Answer from the drawing. Dimensions are ordinates in mm from the lowest x, y and z of the part. A direction names the side the tool comes from. Give positions to 0.01 mm unless a question says otherwise; leave off trailing zeros. Order: outer loops, then holes, each group sorted by start corner. A loop starts at its lowest first (then second) coordinate and runs counter-clockwise, first axis right, second up. Notation, with made-up numbers: (72, 16.5) -> (119, 16.5) arc R16 cw to (119, 41.5) -> close; hole circle Ø4 at (59, 42.5). An arc over 180 degrees is marked (long way). Answer as a JSON object with one key per item and string values. Group by question number.
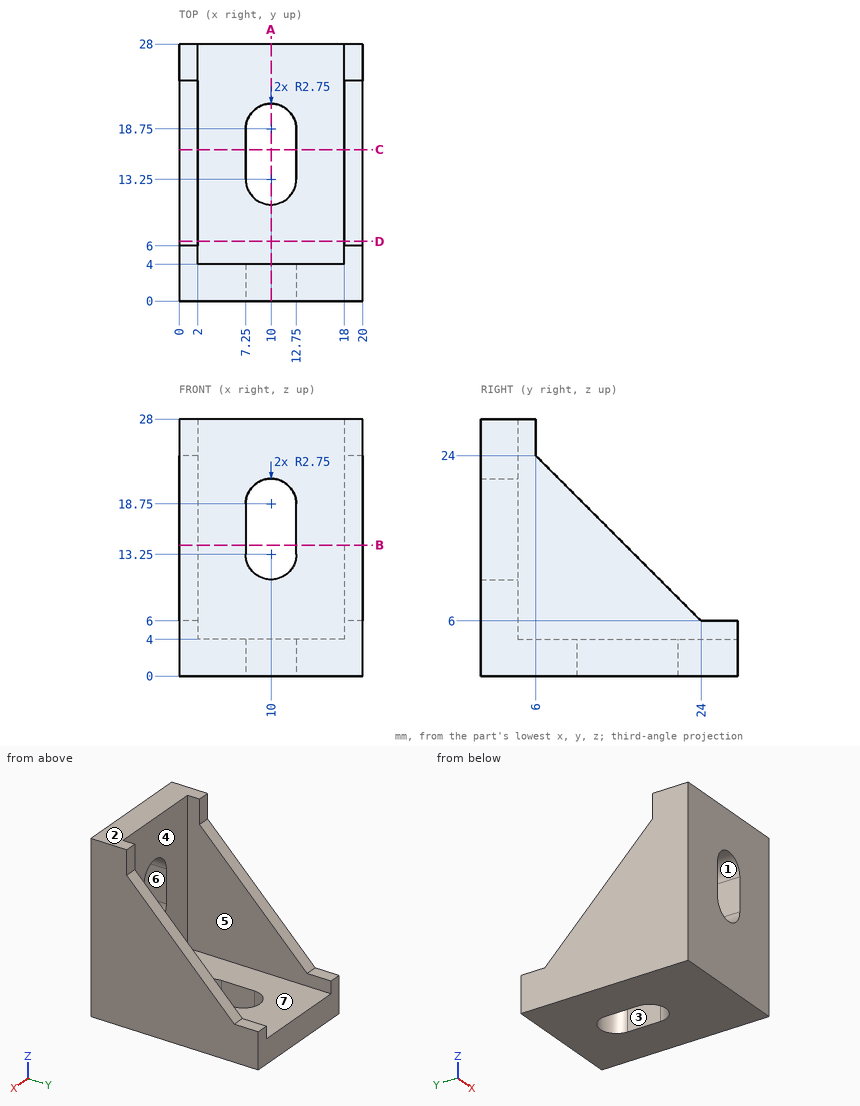
(1) A cutting plane is placed at B-B (z = 14.25). Determine the outline of the cut face in (x, y).
(2) Which of the six approach directions +Z, -Z, +X, -X, +Y, -Y give full straight-line access (tool end or side, diameter ignored) to the marked faces 1, 2, 3 and 4?
(3) Find the intervals of material crossed by line 1 along X through (y, z) = (6.5, 14); line 2 along Y through (x, z) = (5.25, 25.75), in increasing order. Write a range as [from, to].
(4) For a pull along Z with two mould halves and no side action, classify the marked faces 5, 6 and 7 as +Z half, -Z half, draft (parallel to the pull), parting line (faces both ways), or undercut.
(5) Flat-ended cylindrical pins translate along their axes: pin 1 Ø10 at (x, z) = (8, 22.5) entering from +Y; pin 2 Ø2 at (x, y) = (18.5, 25.5) entering from +Z; pin 3 Ø1 at (x, z) = (19, 27) entering from +Y. Find the tip coordinate at first contact, or state that the pin passes through.
(6) A cutting plane is placed at A-A (x = 10). Determine the outline of the cut face in (y, z).
(7) A cutting plane is placed at C-C (y = 16.5). Determine the outline of the cut face in (x, z), and give its area (3 significant figures).
(8) A cutting plane is placed at D-D (y = 6.5). Determine the outline of the cut face in (x, z), and give its area (3 significant figures).
Check sheet entries:
{
 "1": {"outline": "(0, 0) -> (7.25, 0) -> (7.25, 4) -> (2, 4) -> (2, 15.75) -> (0, 15.75) -> close; (12.75, 0) -> (20, 0) -> (20, 15.75) -> (18, 15.75) -> (18, 4) -> (12.75, 4) -> close"},
 "2": {"face 1": "+Y, -Y", "face 2": "+Z, +X, -X, +Y, -Y", "face 3": "+Z, -Z", "face 4": "+Z, +Y"},
 "3": {"line 1": "x = [0, 2], [18, 20]", "line 2": "y = [0, 4]"},
 "4": {"face 5": "draft", "face 6": "undercut", "face 7": "+Z half"},
 "5": {"pin 1": "stops at y = 4", "pin 2": "stops at z = 6", "pin 3": "stops at y = 6"},
 "6": {"outline": "(0, 0) -> (10.5, 0) -> (10.5, 4) -> (4, 4) -> (4, 10.5) -> (0, 10.5) -> close; (0, 21.5) -> (4, 21.5) -> (4, 28) -> (0, 28) -> close; (21.5, 0) -> (28, 0) -> (28, 4) -> (21.5, 4) -> close"},
 "7": {"outline": "(0, 0) -> (7.25, 0) -> (7.25, 4) -> (2, 4) -> (2, 13.5) -> (0, 13.5) -> close; (12.75, 0) -> (20, 0) -> (20, 13.5) -> (18, 13.5) -> (18, 4) -> (12.75, 4) -> close", "area": "96.0 mm2"},
 "8": {"outline": "(0, 0) -> (20, 0) -> (20, 23.5) -> (18, 23.5) -> (18, 4) -> (2, 4) -> (2, 23.5) -> (0, 23.5) -> close", "area": "158 mm2"}
}
